```python
from build123d import *

# Parameters (mm, degrees)
F0_W     = 96.4152663946
F0_H     = 100.6311327219
F1_DEPTH = 1.4986
F3_DEPTH = 96.4152663946


with BuildPart() as f1:
    # F0 (on Front) → F1 (new body)
    with BuildSketch(Plane.XZ):
        Rectangle(F0_W, F0_H)
    extrude(amount=F1_DEPTH)

    # F2 (on face) → F3 (join, through all)
    with BuildSketch(Plane.YZ.offset(48.2076331973)):
        with BuildLine():
            Line((7.7614295296, 51.814166361), (0, 51.814166361))
            ThreePointArc((0, 51.814166361), (-1.0596702223, 51.3752365832), (-1.4986, 50.315566361))
            Line((-1.4986, 50.315566361), (0, 50.315566361))
            Line((0, 50.315566361), (7.6948883943, 50.315566361))
            Line((7.6948883943, 50.315566361), (7.7614295296, 51.814166361))
        make_face()
    extrude(amount=-F3_DEPTH)


solid = f1.part
```
Source: CAD feature listing. Evaluate the final solid. Frame: model axes, mm. A direction names the side the tool comes from. Coordinates: 2 decimals unless noted, no trailing zeros. Write each loop counter-clockwise with the first axis right and the second up, starting at its lowest first coordinate (ties: lowest second). Pieces come first, ordered by that corner, then holes. Notation, with made-up numbers: (25.5, 52) -> (58.5, 52) arc R10 cw to (58.5, 63) -> close; hole circle Ø7 at (76, 23.5). An arc over 180 degrees is marked (long way). Return JSON: item names as keys, results as strings. Group by question number.
1) Contact query for flat-ended pins moving along their axis: P1, Ø6, axis at x = 9, z = 18, coming from the +Y side; P2, Ø2, axis at x = 4.5, y = 1.5, coming from the -Z side. Output: stop coordinate, or through.
2) Section query A-A, the plane x = -23.5. Return loops of the section in (y, z), plus the area to 3 significant figures.
3) Section query B-B, the plane z = -13. Return loops of the section in (x, y), plus the area to 3 significant figures.
4) Ray query, line 1 along Z through (x, y) = (25.5, 1.75); line 2 along Y through (x, z) = (14.5, 10); line 3 along Z through (x, y) = (13.5, -0.25). Return the intervals inside material, ascending.
5) Set-up query: faces 1 (the face through (1, 4, 51.814)), 2 (the face through (-1, 0, 1)). Return all of +Z, -Z, +X, -X, +Y, -Y with unobstructed straight access to the full face (end or side cutting, diameter ignored); none if empty.
6) Section query C-C, the plane y = 4.5. Return loops of the section in (x, z).
From the geometry:
{
 "1": {"P1": "y = 0", "P2": "z = 50.32"},
 "2": {"outline": "(-1.5, -50.32) -> (0, -50.32) -> (0, 50.32) -> (7.69, 50.32) -> (7.76, 51.81) -> (0, 51.81) arc R1.5 ccw to (-1.5, 50.32) -> close", "area": "164 mm²"},
 "3": {"outline": "(-48.21, -1.5) -> (48.21, -1.5) -> (48.21, 0) -> (-48.21, 0) -> close", "area": "144 mm²"},
 "4": {"line 1": "50.32 to 51.81", "line 2": "-1.5 to 0", "line 3": "-50.32 to 51.79"},
 "5": {"face 1": "+Z, +X, -X, +Y, -Y", "face 2": "-Z, +X, -X, +Y"},
 "6": {"outline": "(-48.21, 50.32) -> (48.21, 50.32) -> (48.21, 51.81) -> (-48.21, 51.81) -> close"}
}
